Check sheet for the modelled part. Datum: model origin and axes. Units: mm. Give positions to 0.01 mm unless a question says otherwise; leave off trailing zeros. Order: outer loops, then holes, each group sorted by start corner. A loop starts at its lowest first (then second) coordinate and runs counter-clockwise, first axis right, second up.
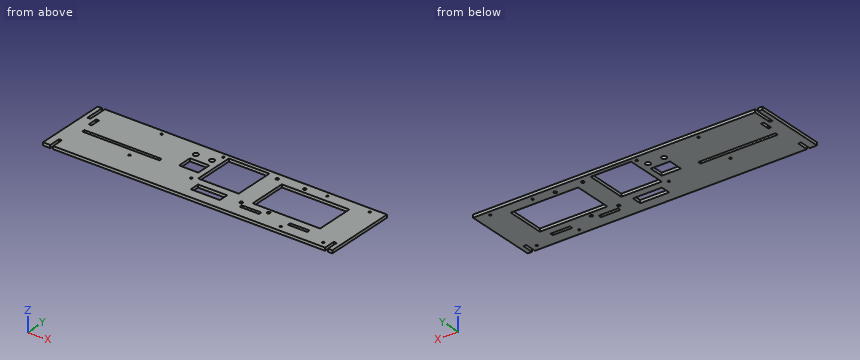
Autodesk Inventor part; units mm, degrees
ref_plane "YZ Plane" through (0, 0, 0) normal (1, 0, 0) x (0, 1, 0)
ref_plane "XZ Plane" through (0, 0, 0) normal (0, 1, 0) x (-1, 0, 0)
ref_plane "XY Plane" through (0, 0, 0) normal (0, 0, 1) x (1, 0, 0)
sketch "Sketch1" plane through (0, 0, 0) normal (0, 0, 1) x (1, 0, 0)
  line L0 (0, 0) -> (300, 0)
  line L1 (300, 0) -> (300, 65)
  line L2 (300, 65) -> (0, 65)
  line L3 (0, 65) -> (0, 0)
  line L4 (0, 0) -> (300, 0)
  line L5 (300, 0) -> (300, -10)
  line L6 (300, -10) -> (0, -10)
  line L7 (0, -10) -> (0, 0)
  dimension "d0" = 300
  dimension "d1" = 65
  dimension "d2" = 10
extrude "Extrusion1" add sketch "Sketch1" along normal blind 3
sketch "Sketch3" plane through (0, 0, 3) normal (0, 0, 1) x (1, 0, 0)
  line L0 (139, 61) -> (181, 61)
  line L1 (181, 61) -> (181, 19)
  line L2 (181, 19) -> (139, 19)
  line L3 (139, 19) -> (139, 61)
  line L4 (139, 61) -> (181, 19) construction
  line L5 (181, 61) -> (139, 19) construction
  line L6 (300, -10) -> (300, 65)
  line L7 (300, 65) -> (0, 65)
  line L8 (0, 65) -> (0, -10)
  line L9 (145, 11) -> (175, 11)
  line L10 (175, 11) -> (175, 1)
  line L11 (175, 1) -> (145, 1)
  line L12 (145, 1) -> (145, 11)
  line L13 (145, 11) -> (175, 1) construction
  line L14 (175, 11) -> (145, 1) construction
  point P0 (0, 0)
  point P1 (160, 40)
  point P2 (160, 6)
  dimension "d12" = 25
  dimension "d13" = 42
  dimension "d14" = 42
  dimension "d19" = 160
  dimension "d57" = 8
  dimension "d58" = 30
  dimension "d59" = 10
extrude "Extrusion2" cut sketch "Sketch3" against normal blind 3
sketch "Sketch2" plane through (0, 0, 3) normal (0, 0, 1) x (1, 0, 0)
  line L0 (0, -10) -> (300, -10)
  line L1 (7.5, -10) -> (10.5, -10)
  line L2 (10.5, -10) -> (10.5, 2)
  line L3 (10.5, 2) -> (7.5, 2)
  line L4 (7.5, 2) -> (7.5, -10)
  line L5 (295.5, -10) -> (292.5, -10)
  line L6 (292.5, -10) -> (292.5, 2)
  line L7 (292.5, 2) -> (295.5, 2)
  line L8 (295.5, 2) -> (295.5, -10)
  line L9 (300, 65) -> (0, 65)
  line L10 (4.5, 65) -> (7.5, 65)
  line L11 (7.5, 65) -> (7.5, 45)
  line L12 (7.5, 45) -> (4.5, 45)
  line L13 (4.5, 45) -> (4.5, 65)
  line L14 (0, 65) -> (0, -10)
  point P0 (0, 0)
  point P1 (294, 2)
  dimension "d6" = 12
  dimension "d7" = 3
  dimension "d8" = 6
  dimension "d9" = 3
  dimension "d53" = 20
  dimension "d54" = 3
  dimension "d88" = 4.5
extrude "Extrusion3" cut sketch "Sketch2" against normal blind 3
sketch "Sketch4" plane through (0, 0, 3) normal (0, 0, 1) x (1, 0, 0)
  line L0 (15.05, 26.95) -> (95.15, 26.95)
  line L1 (95.15, 26.95) -> (95.15, 23.9)
  line L2 (95.15, 23.9) -> (15.05, 23.9)
  line L3 (15.05, 23.9) -> (15.05, 26.95)
  line L4 (12, 47) -> (15.05, 47)
  line L5 (15.05, 47) -> (15.05, 36.95)
  line L6 (15.05, 36.95) -> (12, 36.95)
  line L7 (12, 36.95) -> (12, 47)
  line L8 (0, 65) -> (0, -10)
  circle A0 centre (113.15, 50) radius 2.6
  circle A1 centre (129.8199, 50) radius 2.6
  line L9 (300, 65) -> (7.5, 65)
  line L10 (113.15, 41.95) -> (133.15, 41.95)
  line L11 (133.15, 41.95) -> (133.15, 26.95)
  line L12 (133.15, 26.95) -> (113.15, 26.95)
  line L13 (113.15, 26.95) -> (113.15, 41.95)
  point P0 (0, 0)
  point P1 (139, 19)
  dimension "d20" = 80.1
  dimension "d21" = 3.05
  dimension "d22" = 3.05
  dimension "d23" = 10.05
  dimension "d28" = 12
  dimension "d56" = 18
  dimension "d60" = 10
  dimension "d77" = 5.2
  dimension "d78" = 5.2
  dimension "d79" = 15
  dimension "d80" = 20
  dimension "d81" = 15
  dimension "d82" = 18
extrude "Extrusion4" cut sketch "Sketch4" against normal blind 3
sketch "Sketch5" plane through (0, 0, 3) normal (0, 0, 1) x (1, 0, 0)
  circle A0 centre (191.5, 58) radius 1.55
  circle A1 centre (220, 58) radius 1.55
  circle A2 centre (220, 8.5) radius 1.55
  circle A3 centre (191.5, 8.5) radius 1.55
  line L0 (300, -10) -> (300, 65)
  point P0 (0, 0)
  dimension "d31" = 28.5
  dimension "d32" = 49.5
  dimension "d33" = 3.1
  dimension "d34" = 3.1
  dimension "d35" = 3.1
  dimension "d36" = 3.1
  dimension "d37" = 80
  dimension "d38" = 7
extrude "Extrusion5" cut sketch "Sketch5" against normal blind 3
sketch "Sketch6" plane through (0, 0, 3) normal (0, 0, 1) x (1, 0, 0)
  circle A0 centre (242, 60) radius 1.1
  circle A1 centre (286, 60) radius 1.1
  circle A2 centre (286, -4) radius 1.1
  circle A3 centre (242, -4) radius 1.1
  circle A4 centre (220, 58) radius 1.55
  circle A5 centre (70, 60) radius 1.1
  circle A6 centre (134, 60) radius 1.1
  circle A7 centre (134, 16) radius 1.1
  circle A8 centre (70, 16) radius 1.1
  point P0 (0, 0)
  point P1 (300, 65)
  point P2 (0, 65)
  dimension "d41" = 2.2
  dimension "d42" = 2.2
  dimension "d43" = 2.2
  dimension "d44" = 2.2
  dimension "d45" = 64
  dimension "d46" = 44
  dimension "d50" = 5
  dimension "d51" = 14
  dimension "d61" = 64
  dimension "d62" = 44
  dimension "d63" = 2.2
  dimension "d64" = 2.2
  dimension "d65" = 2.2
  dimension "d66" = 2.2
  dimension "d67" = 70
  dimension "d68" = 5
extrude "Extrusion6" cut sketch "Sketch6" against normal blind 3 contours A0 | A1 | A2 | A3 | A5 | A6 | A7 | A8
sketch "Sketch7" plane through (0, 0, 3) normal (0, 0, 1) x (1, 0, 0)
  line L0 (244.95, 5.05) -> (265, 5.05)
  line L1 (265, 5.05) -> (265, 2)
  line L2 (265, 2) -> (244.95, 2)
  line L3 (244.95, 2) -> (244.95, 5.05)
  line L4 (194.9, 5.05) -> (215, 5.05)
  line L5 (215, 5.05) -> (215, 2)
  line L6 (215, 2) -> (194.9, 2)
  line L7 (194.9, 2) -> (194.9, 5.05)
  line L8 (300, -10) -> (300, 65)
  line L9 (200, 53) -> (270, 53)
  line L10 (270, 53) -> (270, 13)
  line L11 (270, 13) -> (200, 13)
  line L12 (200, 13) -> (200, 53)
  line L13 (300, 65) -> (7.5, 65)
  point P0 (0, 0)
  dimension "d69" = 20.05
  dimension "d70" = 3.05
  dimension "d73" = 20.1
  dimension "d74" = 29.95
  dimension "d75" = 35
  dimension "d76" = 12
  dimension "d83" = 70
  dimension "d84" = 40
  dimension "d85" = 12
  dimension "d86" = 30
extrude "Extrusion7" cut sketch "Sketch7" against normal blind 3
properties part number "2ndSideboard"
1) Section check B-B, the plane x = 81.5. Record the cut outline in (y, z), then the cut area to 3 significant figures.
Recorded:
outline: (-10, 0) - (23.9, 0) - (23.9, 3) - (-10, 3) - close; (26.95, 0) - (65, 0) - (65, 3) - (26.95, 3) - close
area: 216 mm2
2) Material ranges on L1, parallel to Y at x = 286, z = 1.5; L2, parallel to X at y = 31, z = 0.6; L3, parallel to Y at x = 134, z = 1.1, recorded low to high.
Recorded:
L1: y = -10 to -5.1, -2.9 to 58.9, 61.1 to 65
L2: x = 0 to 113.15, 133.15 to 139, 181 to 200, 270 to 300
L3: y = -10 to 14.9, 17.1 to 58.9, 61.1 to 65
3) Depth check by flat-ended pin: pin 1 Ø1.3 at (x, y) = (286, 60) entering from -Z. Enter the tip coordinate at first touch or a pass-through.
Recorded:
pin 1: passes through
4) Section check C-C, the plane z = 2.05. State how many separate pieces and enclosed holes the cut face has, then the cut area to 3 significant figures.
Recorded:
separate pieces: 1
enclosed holes: 22
area: 16,700 mm2
5) Section check A-A, the plane x = 229. Record the cut outline in (y, z).
Recorded:
outline: (-10, 0) - (13, 0) - (13, 3) - (-10, 3) - close; (53, 0) - (65, 0) - (65, 3) - (53, 3) - close
